Autodesk Inventor part; units mm, degrees
ref_plane "YZ Plane" through (0, 0, 0) normal (1, 0, 0) x (0, 1, 0)
ref_plane "XZ Plane" through (0, 0, 0) normal (0, 1, 0) x (-1, 0, 0)
ref_plane "XY Plane" through (0, 0, 0) normal (0, 0, 1) x (1, 0, 0)
sketch "スケッチ1" plane through (0, 0, 0) normal (0, 1, 0) x (-1, 0, 0)
  circle A0 centre (0, 0) radius 2.75
  dimension "d0" = 5.5
extrude "押し出し1" add sketch "スケッチ1" along normal blind 3
sketch "スケッチ2" plane through (0, 0, 0) normal (0, -1, 0) x (1, 0, 0)
  circle A0 centre (0, 0) radius 1.5
  dimension "d3" = 3
extrude "押し出し2" add sketch "スケッチ2" along normal blind 4
fillet "フィレット1" radius 0.5 1 edges at (2.75, 3, 0)
fillet "フィレット1" radius 0.2 1 edges at (2.75, 0, 0)
sketch "スケッチ3" plane through (0, 3, 0) normal (0, 1, 0) x (1, 0, 0)
  line L0 (0, 1.4434) -> (-1.25, 0.7217)
  line L1 (-1.25, 0.7217) -> (-1.25, -0.7217)
  line L2 (-1.25, -0.7217) -> (0, -1.4434)
  line L3 (0, -1.4434) -> (1.25, -0.7217)
  line L4 (1.25, -0.7217) -> (1.25, 0.7217)
  line L5 (1.25, 0.7217) -> (0, 1.4434)
  line L6 (0, 1.4434) -> (0, -1.4434) construction
  circle A0 centre (0, 0) radius 1.4434 construction
  dimension "d12" = 2.5
extrude "押し出し3" cut sketch "スケッチ3" against normal blind 2
thread "ねじ1"
properties part number "M3-CapScrew"
Input: part model. Units: mm. Frame: model coordinates. A direction names the side the tool comes from. Round coordinates to 2 decimals unless told otherwise and drop trailing zeros. Loops run counter-clockwise (first coordinate to the right, second up) from the corner with the lowest first, then second, coordinate; pieces in that order, holes last. Notation, with made-up numbers: M -4.75,50.25 L 21.25,50.25 A20 ccw 21.25,70.25 Z; hole C 35,-34.5 d5. An arc over 180 degrees is marked long. Answer as CSV lines item,"result". Start each with the question number.
(1) Section C-C, the plane y = -3. Output: boundary loops of the cut face in (x, z), plus the area to 3 significant figures.
(2) Section D-D, the plane y = 0.5. Output: boundary loops of the cut face in (x, z).
(3) Line query: line 1 (Y direction, x = 0.55, z = 0.85); line 2 (Y direction, x = 2.1, z = -0.05); line 3 (X direction, y = 2.5, z = -1). Output: solid intervals per line, ascending. Write a range as [from, to].
(4) Section B-B, the plane y = 2.75. Output: boundary loops of the cut face in (x, z).
(5) Draft query along X for faces 4 (the cylindrical face through (0.596, 1.334, 2.685)), 5 (the flat face through (-1.5, 3, 0)), 6 (the flat face through (-0.616, 2.014, -1.088)). Return one class per face: released by +X, released by -X, zero draft, split by the parting line, or undercut.
(6) Section A-A, the plane z = 0. Output: boundary loops of the cut face in (x, y), plus the area to 3 significant figures.
(7) Reachability of faces 1 (the cylindrical face through (-1.5, -1.97, -0.07)), 2 (the flat face through (0.616, 2.014, 1.088)), 3 (the flat face through (0, -4, 0)) from +Z, -Z, +X, -X, +Y, -Y: full face, straight path, thin tool, end or side. Return the list, or none.
(8) First-contact query: pin 1 (1.5 mm diameter, centred on x = -1.5, y = 1.5, fed in from +Z). Flat tip, straight axial feed; report the tip coordinate or a pass-through.
Values found:
1,outline,"C 0,0 d3"
1,area,"7.07 mm²"
2,outline,"C 0,0 d5.5"
3,line 1,"y = [-4, 1]"
3,line 2,"y = [0, 3]"
3,line 3,"x = [-2.56, -0.77], [0.77, 2.56]"
4,outline,"C 0,0 d5.37; hole M -1.25,-0.72 L 0,-1.44 L 1.25,-0.72 L 1.25,0.72 L 0,1.44 L -1.25,0.72 Z"
5,face 4,"split by the parting line"
5,face 5,"zero draft"
5,face 6,"undercut"
6,outline,"M -2.75,0.2 A0.2 ccw -2.55,0 L -1.5,0 L -1.5,-4 L 1.5,-4 L 1.5,0 L 2.55,0 A0.2 ccw 2.75,0.2 L 2.75,2.5 A0.5 ccw 2.25,3 L 1.25,3 L 1.25,1 L -1.25,1 L -1.25,3 L -2.25,3 A0.5 ccw -2.75,2.5 Z"
6,area,"23.4 mm²"
7,face 1,"-Y"
7,face 2,"+Y"
7,face 3,"+Z, -Z, +X, -X, -Y"
8,pin 1,"stops at z = 2.65"
